Can you work these out from the model? Positions are in its coordinate system, mm. A direction names the side the tool comes from. Give positions to 0.01 mm unless a question says otherwise; leave off trailing zeros. Loops run counter-clockwise (first coordinate to the right, second up) from the corner with the lowest first, then second, coordinate; pieces in that order, holes last. Notation, with made-up numbers: M 21,-32.75 L 66,-32.75 A25 ccw 66,3.25 Z; hole C -29,25 d4. An arc over 180 degrees is marked long. Answer as a JSON object with one key per item and string values.
```python
from build123d import *

# Parameters (mm, degrees)
SKETCH1_W           = 120
SKETCH1_H           = 35
BOSS_EXTRUDE1_DEPTH = 5
CUT_EXTRUDE1_DEPTH  = 3
SKETCH5_W           = 28
SKETCH5_H           = 20
CUT_EXTRUDE2_DEPTH  = 3
CHAMFER1_SIZE       = 4
SKETCH6_R           = 8
CUT_EXTRUDE3_DEPTH  = 5
SKETCH7_R           = 2
CUT_EXTRUDE4_DEPTH  = 5
CUT_EXTRUDE5_DEPTH  = 5
SKETCH9_W           = 85
SKETCH9_H           = 3
BOSS_EXTRUDE2_DEPTH = 50
SKETCH10_W          = 85
SKETCH10_H          = 4
BOSS_EXTRUDE3_DEPTH = 32
BOSS_EXTRUDE4_DEPTH = 50
SKETCH12_R          = 17.5
BOSS_EXTRUDE5_DEPTH = 4
SKETCH13_R          = 5
SKETCH13_R_2        = 4
CUT_EXTRUDE6_DEPTH  = 4
BOSS_EXTRUDE6_DEPTH = 14
SKETCH15_R          = 15.5
CUT_EXTRUDE7_DEPTH  = 46
SKETCH16_R          = 3.5
CUT_EXTRUDE8_DEPTH  = 2
SKETCH17_R          = 2
CUT_EXTRUDE9_DEPTH  = 15
BOSS_EXTRUDE7_REACH = 52
SKETCH18_R          = 4
SKETCH19_R          = 2
CUT_EXTRUDE10_DEPTH = 20
CUT_EXTRUDE10_TAPER = 3


with BuildPart() as part:
    # Sketch1 → Boss-Extrude1 (new body)
    with BuildSketch(Plane.XY):
        Rectangle(SKETCH1_W, SKETCH1_H)
    extrude(amount=BOSS_EXTRUDE1_DEPTH)

    # Sketch4 → Cut-Extrude1 (cut)
    with BuildSketch(Plane.XY.offset(5)):
        with BuildLine():
            Line((15, -11.5), (45, -11.5))
            Line((45, -11.5), (53.093205875, -4.710922816))
            ThreePointArc((53.093205875, -4.710922816), (55.688146307, -0.852928933), (54.400122175, 3.614601312))
            Line((54.400122175, 3.614601312), (45, 11.5))
            Line((45, 11.5), (15, 11.5))
            Line((15, 11.5), (7.291284487, 4.451783997))
            ThreePointArc((7.291284487, 4.451783997), (5.029380926, 0.301948581), (6.822687206, -4.07085307))
            Line((6.822687206, -4.07085307), (15, -11.5))
        make_face()
    extrude(amount=-CUT_EXTRUDE1_DEPTH, mode=Mode.SUBTRACT)

    # Sketch5 → Cut-Extrude2 (cut)
    with BuildSketch(Plane.XY.offset(2)):
        with Locations((30, 0)):
            Rectangle(SKETCH5_W, SKETCH5_H)
    extrude(amount=-CUT_EXTRUDE2_DEPTH, mode=Mode.SUBTRACT)

    # Chamfer1
    chamfer1_edges = [part.edges().sort_by_distance(p)[0] for p in [
        (44, 10, 1),
        (16, 10, 1),
    ]]
    chamfer(chamfer1_edges, length=CHAMFER1_SIZE)

    # Sketch6 → Cut-Extrude3 (cut)
    with BuildSketch(Plane.XY.offset(5)):
        with Locations((-15, 0)):
            Circle(SKETCH6_R)
        with Locations((-45, 0)):
            Circle(SKETCH6_R)
    extrude(amount=-CUT_EXTRUDE3_DEPTH, mode=Mode.SUBTRACT)

    # Sketch7 → Cut-Extrude4 (cut)
    with BuildSketch(Plane.XY.offset(2)):
        with Locations((11.038079628, 0)):
            Circle(SKETCH7_R)
        with Locations((48.961920372, 0)):
            Circle(SKETCH7_R)
    extrude(amount=-CUT_EXTRUDE4_DEPTH, mode=Mode.SUBTRACT)

    # Sketch8 → Cut-Extrude5 (cut)
    with BuildSketch(Plane.XY.offset(5)):
        with BuildLine():
            Line((-60, 17.5), (-60, -6.7e-08))
            ThreePointArc((-60, -6.7e-08), (-54.874368695, 12.374368647), (-42.5, 17.5))
            Line((-42.5, 17.5), (-60, 17.5))
        make_face()
        with BuildLine():
            Line((-60, -17.5), (-42.5, -17.5))
            ThreePointArc((-42.5, -17.5), (-54.874368647, -12.374368695), (-60, -6.7e-08))
            Line((-60, -6.7e-08), (-60, -17.5))
        make_face()
        with BuildLine():
            ThreePointArc((42.5, 17.5), (54.874368671, 12.374368671), (60, 0))
            Line((60, 0), (60, 17.5))
            Line((60, 17.5), (42.5, 17.5))
        make_face()
        with BuildLine():
            Line((42.5, -17.5), (60, -17.5))
            Line((60, -17.5), (60, 0))
            ThreePointArc((60, 0), (54.874368671, -12.374368671), (42.5, -17.5))
        make_face()
    extrude(amount=-CUT_EXTRUDE5_DEPTH, mode=Mode.SUBTRACT)

    # Sketch9 → Boss-Extrude2 (add)
    with BuildSketch(Plane(origin=(0, 0, 0), x_dir=(-1, 0, 0), z_dir=(0, 0, -1))):
        with Locations((0, -16)):
            Rectangle(SKETCH9_W, SKETCH9_H)
    extrude(amount=BOSS_EXTRUDE2_DEPTH)

    # Sketch10 → Boss-Extrude3 (add)
    with BuildSketch(Plane(origin=(0, -14.5, 0), x_dir=(1, 0, 0), z_dir=(0, 1, 0))):
        with Locations((0, 48)):
            Rectangle(SKETCH10_W, SKETCH10_H)
    extrude(amount=BOSS_EXTRUDE3_DEPTH)

    # Sketch11 → Boss-Extrude4 (add)
    with BuildSketch(Plane(origin=(0, 0, 0), x_dir=(-1, 0, 0), z_dir=(0, 0, -1))):
        with BuildLine():
            Line((42.5, 17.5), (42.5, 15.5))
            ThreePointArc((42.5, 15.5), (58, 0), (42.5, -15.5))
            Line((42.5, -15.5), (42.5, -17.5))
            ThreePointArc((42.5, -17.5), (60, 0), (42.5, 17.5))
        make_face()
        with BuildLine():
            Line((-42.5, 17.5), (-42.5, 15.5))
            ThreePointArc((-42.5, 15.5), (-58, 0), (-42.5, -15.5))
            Line((-42.5, -15.5), (-42.5, -17.5))
            ThreePointArc((-42.5, -17.5), (-60, 0), (-42.5, 17.5))
        make_face()
    extrude(amount=BOSS_EXTRUDE4_DEPTH)

    # Sketch12 → Boss-Extrude5 (add)
    with BuildSketch(Plane(origin=(0, 0, -50), x_dir=(-1, 0, 0), z_dir=(0, 0, -1))):
        with Locations((-42.5, 0)):
            Circle(SKETCH12_R)
        with Locations((42.5, 0)):
            Circle(SKETCH12_R)
    extrude(amount=-BOSS_EXTRUDE5_DEPTH)

    # Sketch13 → Cut-Extrude6 (cut)
    with BuildSketch(Plane(origin=(0, 0, -50), x_dir=(-1, 0, 0), z_dir=(0, 0, -1))):
        with Locations((-30, -2)):
            Circle(SKETCH13_R)
        with Locations((30, 0)):
            Circle(SKETCH13_R_2)
    extrude(amount=-CUT_EXTRUDE6_DEPTH, mode=Mode.SUBTRACT)

    # Sketch14 → Boss-Extrude6 (add)
    with BuildSketch(Plane(origin=(0, 17.5, 0), x_dir=(1, 0, 0), z_dir=(0, 1, 0))):
        with BuildLine():
            Line((-42.5, 14.5), (-67.5, 14.5))
            ThreePointArc((-67.5, 14.5), (-75.5, 22.5), (-67.5, 30.5))
            Line((-67.5, 30.5), (-42.5, 30.5))
            Line((-42.5, 30.5), (-42.5, 14.5))
        make_face()
        with BuildLine():
            Line((42.5, 30.5), (67.5, 30.5))
            ThreePointArc((67.5, 30.5), (75.5, 22.5), (67.5, 14.5))
            Line((67.5, 14.5), (42.5, 14.5))
            Line((42.5, 14.5), (42.5, 30.5))
        make_face()
    extrude(amount=-BOSS_EXTRUDE6_DEPTH)

    # Sketch15 → Cut-Extrude7 (cut)
    with BuildSketch(Plane(origin=(0, 0, 0), x_dir=(-1, 0, 0), z_dir=(0, 0, -1))):
        with Locations((-42.5, 0)):
            Circle(SKETCH15_R)
        with Locations((42.5, 0)):
            Circle(SKETCH15_R)
    extrude(amount=CUT_EXTRUDE7_DEPTH, mode=Mode.SUBTRACT)

    # Sketch16 → Cut-Extrude8 (cut)
    with BuildSketch(Plane.XZ.offset(-3.5)):
        with Locations((67.5, -22.5)):
            Circle(SKETCH16_R)
        with Locations((-67.5, -22.5)):
            Circle(SKETCH16_R)
    extrude(amount=-CUT_EXTRUDE8_DEPTH, mode=Mode.SUBTRACT)

    # Sketch17 → Cut-Extrude9 (cut, through all)
    with BuildSketch(Plane.XZ.offset(-3.5)):
        with Locations((-67.5, -22.5)):
            Circle(SKETCH17_R)
        with Locations((67.5, -22.5)):
            Circle(SKETCH17_R)
    extrude(amount=-CUT_EXTRUDE9_DEPTH, mode=Mode.SUBTRACT)

    # Sketch18 → Boss-Extrude7 (add, up to next)
    with BuildSketch(Plane(origin=(0, 0, 0), x_dir=(-1, 0, 0), z_dir=(0, 0, -1)), mode=Mode.PRIVATE) as boss_extrude7_sk1:
        with Locations((-48.961920372, 0)):
            Circle(SKETCH18_R)
    boss_extrude7_tool1 = extrude(boss_extrude7_sk1.sketch, amount=BOSS_EXTRUDE7_REACH, mode=Mode.PRIVATE) - part.part
    add(boss_extrude7_tool1.solids().sort_by_distance((48.96192, 0, 0))[0])
    # Sketch18 → Boss-Extrude7 (add, up to next)
    with BuildSketch(Plane(origin=(0, 0, 0), x_dir=(-1, 0, 0), z_dir=(0, 0, -1)), mode=Mode.PRIVATE) as boss_extrude7_sk2:
        with Locations((-11.038079628, 0)):
            Circle(SKETCH18_R)
    boss_extrude7_tool2 = extrude(boss_extrude7_sk2.sketch, amount=BOSS_EXTRUDE7_REACH, mode=Mode.PRIVATE) - part.part
    add(boss_extrude7_tool2.solids().sort_by_distance((11.03808, 0, 0))[0])

    # Sketch19 → Cut-Extrude10 (cut)
    with BuildSketch(Plane.XY):
        with Locations((11.038079628, 0)):
            Circle(SKETCH19_R)
        with Locations((48.961920372, 0)):
            Circle(SKETCH19_R)
    extrude(amount=-CUT_EXTRUDE10_DEPTH, taper=CUT_EXTRUDE10_TAPER, mode=Mode.SUBTRACT)


solid = part.part
```
1) For faces 1 (the flat face through (61, 12, -14.5)), 2 (the flat face through (59, 17.5, -23)), 3 (the cylindrical face through (-70.08, 4.486, -20.135)), 4 (the flat face through (30, 11.5, 4)), 5 (the flat face through (-1, 1, -46)), which set-ups out of +Z, -Z, +X, -X, +Y, -Y let a thin tool reach every point of the face, with its end or its side?
Answer list:
{"face 1": "+Z, +X, +Y", "face 2": "+Z, -Z, +X, -X, +Y", "face 3": "-Y", "face 4": "+Z", "face 5": "none"}
2) Suppose I cut it at C-C, the plane x = 30. Write out the boundary of the cut face in (y, z).
Answer list:
{"outline": "M -17.5,-50 L -7,-50 L -7,-46 L -14.5,-46 L -14.5,0 L -10,0 L -10,2 L -11.5,2 L -11.5,5 L -17.5,5 Z; M 3,-50 L 17.5,-50 L 17.5,-46 L 3,-46 Z; M 10,0 L 17.5,0 L 17.5,5 L 11.5,5 L 11.5,2 L 10,2 Z"}
3) If we mould it in two halves opening along Y, with no side actions, what happens to faces 6 (the conical face through (50.32, -0.56, -10.14)), 7 (the flat face through (-1, 17.5, -48)), 8 (the cylindrical face through (75.498, 10.598, -22.676)), 9 (the flat face through (-1, 1, 0))? For each: +Y half, -Y half, draft (parallel to the pull), parting line (faces both ways), or undercut.
Answer list:
{"face 6": "undercut", "face 7": "+Y half", "face 8": "draft", "face 9": "undercut"}
4) Suppose I cut it at B-B, the plane z = -38. Write out the boundary of the cut face in (x, y), and give its area (3 significant figures).
Answer list:
{"outline": "M -42.5,-17.5 L 42.5,-17.5 A17.5 ccw 42.5,17.5 L 42.5,15.5 A15.5 cw long 37.02,-14.5 L -37.02,-14.5 A15.5 cw long -42.5,15.5 L -42.5,17.5 A17.5 ccw Z; C 11.04,0 d8; C 48.96,0 d8", "area": "556 mm^2"}
5) Suppose I cut it at D-D, the plane z = -3. Write out the boundary of the cut face in (x, y), and give its area (3 significant figures).
Answer list:
{"outline": "M -42.5,-17.5 L 42.5,-17.5 A17.5 ccw 42.5,17.5 L 42.5,15.5 A15.5 cw long 37.02,-14.5 L -37.02,-14.5 A15.5 cw long -42.5,15.5 L -42.5,17.5 A17.5 ccw Z; C 11.04,0 d8; C 48.96,0 d8; hole C 11.04,0 d3.69; hole C 48.96,0 d3.69", "area": "534 mm^2"}
6) Please list where these lines run through material, in increasing order: line 1 along Y through (x, z) = (-30, -47.7); line 2 along Y through (x, z) = (30, -47.2); line 3 along X through (y, z) = (11, -22). Write a range as from..to.
Answer list:
{"line 1": "-17.5..-4, 4..17.5", "line 2": "-17.5..-7, 3..17.5", "line 3": "-75.48..-69.44, -65.56..-53.42, 53.42..65.56, 69.44..75.48"}
7) Will these pins go through, and if not, where does the flat tip stop? pin 1 Ø8 at (y, z) = (-1, -27.5) entering from -X; pin 2 Ø6 at (y, z) = (5, -29) entering from +X; pin 3 Ø1.6 at (y, z) = (16.5, -32) entering from +X; pin 4 Ø11 at (x, y) = (59, 9) entering from -Z.
Answer list:
{"pin 1": "x = -60", "pin 2": "x = 74.69", "pin 3": "x = 50.23", "pin 4": "z = -50"}
8) Suppose I cut it at A-A, the plane x = -30. Write out the boundary of the cut face in (y, z).
Answer list:
{"outline": "M -17.5,-50 L -4,-50 L -4,-46 L -14.5,-46 L -14.5,0 L 17.5,0 L 17.5,5 L -17.5,5 Z; M 4,-50 L 17.5,-50 L 17.5,-46 L 4,-46 Z"}
